For this review, take the finished solid that the model builds, in its own axes (mm). Face numbers are marked on the shaded views. Coordinates: 2 decimals unless noted, no trailing zeros. Loops run counter-clockwise (first coordinate to the right, second up) from the corner with the lowest first, then second, coordinate; pieces in that order, holes last. Notation, with made-up numbers: M 44.25,64.25 L 61.25,64.25 A19 cw 61.25,91.25 Z; hole C 10,-0.75 d7. An arc over 180 degrees is marked long. Answer as a JSON object with one key per item and string values. Group by question number.
Item 1: Mouldability with a two-part tool opening along X and no side actions: class the marked faces 1 and 2 as +X half, -X half, draft (parallel to the pull), parting line (faces both ways), or undercut.
Item 2: Add section C-C (x = -25). State the section outline as (y, z) points.
Item 3: Insertion check: pin 1 (6 mm diameter, centred on x = 26.75, y = 375, fed in from +Z); pin 2 (4.5 mm diameter, centred on x = 26.75, y = 525, fed in from +Z). Each pin has a flat end and moves straight along its axis. Give the tip position at first contact, or say it passes through.
Item 4: Add section A-A (z = 10.5). State the section outline as (x, y) points, then the cut area to 3 significant figures.
Item 5: Add section B-B (y = 871). State the section outline as (x, z) points.
Item 6: Wall thickness on L1, parallel to X at y = 349.5, z = -23.5; L2, parallel to X at y = 675, z = -33; L3, parallel to Z at x = -42, y = 959: over which ranges is each line inside the solid? List them lowest first. Write a range as from..to.
from build123d import *

# Parameters (mm, degrees)
BOSS_EXTRUDE1_DEPTH = 1500
SKETCH2_R           = 2
CUT_EXTRUDE1_DEPTH  = 6
SKETCH3_R           = 2.5
CUT_EXTRUDE2_DEPTH  = 6


with BuildPart() as part:
    # Sketch1 → Boss-Extrude1 (new body)
    with BuildSketch(Plane(origin=(0, 0, 0), x_dir=(1, 0, 0), z_dir=(0, 1, 0))):
        Polygon((-75, 35), (-75, -35), (-69, -35), (-69, 29), (69, 29), (69, -35), (75, -35), (75, 35), align=None)
    extrude(amount=BOSS_EXTRUDE1_DEPTH)

    # Sketch2 → Cut-Extrude1 (cut)
    with BuildSketch(Plane(origin=(75, 0, 0), x_dir=(0, 0, -1), z_dir=(1, 0, 0))):
        with Locations((-25, 312.5)):
            Circle(SKETCH2_R)
        with Locations((-25, 287.5)):
            Circle(SKETCH2_R)
        with Locations((-25, 587.5)):
            Circle(SKETCH2_R)
        with Locations((-25, 612.5)):
            Circle(SKETCH2_R)
        with Locations((-25, 1212.5)):
            Circle(SKETCH2_R)
        with Locations((-25, 1187.5)):
            Circle(SKETCH2_R)
        with Locations((-25, 887.5)):
            Circle(SKETCH2_R)
        with Locations((-25, 912.5)):
            Circle(SKETCH2_R)
    extrude(amount=-CUT_EXTRUDE1_DEPTH, mode=Mode.SUBTRACT)

    # Sketch3 → Cut-Extrude2 (cut)
    with BuildSketch(Plane(origin=(0, 0, -35), x_dir=(-1, 0, 0), z_dir=(0, 0, -1))):
        with Locations((-26.75, 75)):
            Circle(SKETCH3_R)
        with Locations((-26.75, 225)):
            Circle(SKETCH3_R)
        with Locations((-26.75, 375)):
            Circle(SKETCH3_R)
        with Locations((-26.75, 525)):
            Circle(SKETCH3_R)
        with Locations((-26.75, 675)):
            Circle(SKETCH3_R)
        with Locations((-26.75, 825)):
            Circle(SKETCH3_R)
        with Locations((-26.75, 975)):
            Circle(SKETCH3_R)
        with Locations((-26.75, 1125)):
            Circle(SKETCH3_R)
        with Locations((-26.75, 1275)):
            Circle(SKETCH3_R)
        with Locations((-26.75, 1425)):
            Circle(SKETCH3_R)
    extrude(amount=-CUT_EXTRUDE2_DEPTH, mode=Mode.SUBTRACT)


solid = part.part
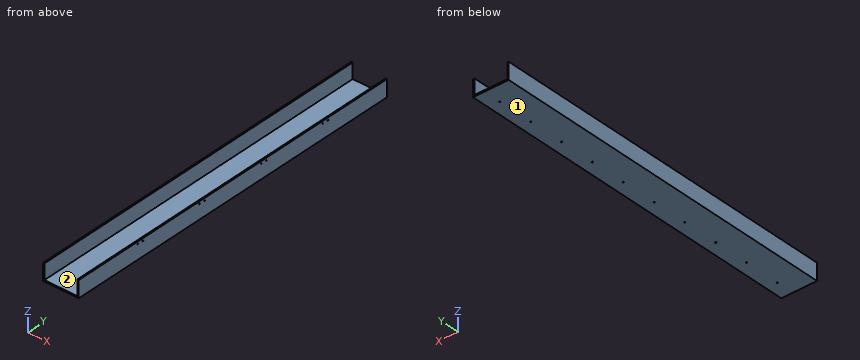
From the geometry:
{
 "1": {"face 1": "draft", "face 2": "undercut"},
 "2": {"outline": "M 0,-35 L 1500,-35 L 1500,-29 L 0,-29 Z"},
 "3": {"pin 1": "stops at z = -29", "pin 2": "passes through"},
 "4": {"outline": "M -75,0 L -69,0 L -69,1500 L -75,1500 Z; M 69,0 L 75,0 L 75,1500 L 69,1500 Z", "area": "18,000 mm²"},
 "5": {"outline": "M -75,-35 L 75,-35 L 75,35 L 69,35 L 69,-29 L -69,-29 L -69,35 L -75,35 Z"},
 "6": {"L1": "x = -75..-69, 69..75", "L2": "x = -75..24.25, 29.25..75", "L3": "z = -35..-29"}
}
